For this review, take the finished solid that the model builds, in its own axes (mm). A direction names the side the tool comes from. Coordinates: 2 decimals unless noted, no trailing zeros. Loops run counter-clockwise (first coordinate to the right, second up) from the corner with the lowest first, then second, coordinate; pieces in that order, holes last. Notation, with made-up numbers: (-28, 48) -> (-7, 48) arc R23 cw to (-7, 83) -> close; hole circle Ø8 at (1.5, 75.25). An arc over 180 degrees is marked (long way). Answer in a Markdown table with one row per item.
from build123d import *

# Parameters (mm, degrees)
SKETCH1_W                 = 45
SKETCH1_H                 = 12.2
BASE_EXTRUDE_DEPTH        = 50
SKETCH16_W                = 33
SKETCH16_H                = 100
TABLE_EXTENSION_DEPTH     = 12.2
SKETCH3_R                 = 2.5
MOUNTHOLES_DEPTH          = 8
SKETCH14_W                = 2.9
SKETCH14_H                = 28.5
CONNECTION_DEPTH          = 44
SKETCH15_R                = 9.95
PISTON_DEPTH              = 72
SKETCH17_W                = 9
SKETCH17_H                = 0.5
SKETCH17_W_2              = 18
GROOVES_DEPTH             = 138.879557948
ENDLOCKPLATE1_DEPTH       = 9
ENDLOCKPLATE2_DEPTH       = 8
SKETCH20_R                = 2
ENDLOCKHOLES_DEPTH        = 117.232751409
SKETCH21_R                = 1.5
ENDLOCKADJUSTSCREWS_DEPTH = 2
SKETCH23_R                = 2
ENDLOCKMOUNTSCREWS_DEPTH  = 2
CHAMFER1_SIZE             = 0.3


with BuildPart() as part:
    # Sketch1 → Base-Extrude (new, symmetric)
    with BuildSketch(Plane.XY):
        Rectangle(SKETCH1_W, SKETCH1_H)
    extrude(amount=BASE_EXTRUDE_DEPTH, both=True)

    # Sketch16 → Table_Extension (add)
    with BuildSketch(Plane(origin=(0, 6.1, 0), x_dir=(-1, 0, 0), z_dir=(0, 1, 0))):
        with Locations((39, 0)):
            Rectangle(SKETCH16_W, SKETCH16_H)
    extrude(amount=-TABLE_EXTENSION_DEPTH)

    # Sketch3 → MountHoles (cut)
    with BuildSketch(Plane(origin=(0, 6.1, 0), x_dir=(-1, 0, 0), z_dir=(0, 1, 0))):
        with Locations(Location((32, -25, 0), (0, 0, 90))):
            Circle(SKETCH3_R)
        with Locations(Location((-8, -25, 0), (0, 0, 270))):
            Circle(SKETCH3_R)
        with Locations(Location((32, 25, 0), (0, 0, 270))):
            Circle(SKETCH3_R)
        with Locations(Location((-8, 25, 0), (0, 0, 90))):
            Circle(SKETCH3_R)
    extrude(amount=-MOUNTHOLES_DEPTH, mode=Mode.SUBTRACT)

    # Sketch14 → Connection (add, symmetric)
    with BuildSketch(Plane.XY):
        with Locations((0, -8.15)):
            Rectangle(SKETCH14_W, SKETCH14_H)
    extrude(amount=CONNECTION_DEPTH, both=True)

    # Sketch15 → Piston (add, symmetric)
    with BuildSketch(Plane.XY):
        with Locations((0, -22.4)):
            Circle(SKETCH15_R)
    extrude(amount=PISTON_DEPTH, both=True)

    # Sketch17 → Grooves (cut, through all)
    with BuildSketch(Plane.XY.offset(50)):
        with Locations((-51, 5.85)):
            Rectangle(SKETCH17_W, SKETCH17_H)
        with Locations((-13.5, 5.85)):
            Rectangle(SKETCH17_W_2, SKETCH17_H)
    extrude(amount=-GROOVES_DEPTH, mode=Mode.SUBTRACT)

    # Sketch18 → EndLockPlate1 (add, symmetric)
    with BuildSketch(Plane(origin=(-39, 0, 0), x_dir=(0, 0, -1), z_dir=(1, 0, 0))):
        Polygon((-50, 5.8), (-52, 5.8), (-52, -1.4), (-78, -1.4), (-78, -3.4), (-50, -3.4), align=None)
    endlockplate1 = extrude(amount=ENDLOCKPLATE1_DEPTH, both=True)

    # Sketch19 → EndLockPlate2 (add, symmetric)
    with BuildSketch(Plane(origin=(-39, 0, 0), x_dir=(0, 0, -1), z_dir=(1, 0, 0))):
        Polygon((-58, -1.4), (-58, -0.4), (-97, -0.4), (-97, -4.5), (-95.6, -5.9), (-78, -5.9), (-78, -1.4), align=None)
    endlockplate2 = extrude(amount=ENDLOCKPLATE2_DEPTH, both=True)

    # Sketch20 → EndLockHoles (cut, through all)
    with BuildSketch(Plane(origin=(0, -0.4, 0), x_dir=(-1, 0, 0), z_dir=(0, 1, 0))):
        with Locations(Location((39, 87.5, 0), (0, 0, 90))):
            Circle(SKETCH20_R)
        with BuildLine():
            Line((32.8, 63), (32.8, 69))
            ThreePointArc((32.8, 69), (33.8, 70), (34.8, 69))
            Line((34.8, 69), (34.8, 63))
            ThreePointArc((34.8, 63), (33.8, 62), (32.8, 63))
        make_face()
        with BuildLine():
            Line((43.2, 69), (43.2, 63))
            ThreePointArc((43.2, 63), (44.2, 62), (45.2, 63))
            Line((45.2, 63), (45.2, 69))
            ThreePointArc((45.2, 69), (44.2, 70), (43.2, 69))
        make_face()
    endlockholes = extrude(amount=-ENDLOCKHOLES_DEPTH, mode=Mode.SUBTRACT)

    # Sketch21 → EndLockAdjustScrews (add)
    with BuildSketch(Plane(origin=(0, -0.4, 0), x_dir=(-1, 0, 0), z_dir=(0, 1, 0))):
        with Locations(Location((44.2, 69, 0), (0, 0, 228.189685104))):
            Circle(SKETCH21_R)
        with Locations(Location((33.8, 69, 0), (0, 0, 228.189685104))):
            Circle(SKETCH21_R)
    endlockadjustscrews = extrude(amount=ENDLOCKADJUSTSCREWS_DEPTH)

    # Sketch23 → EndLockMountScrews (add)
    with BuildSketch(Plane.XY.offset(52)):
        with Locations(Location((-44.2, 2.7, 0), (0, 0, 180))):
            Circle(SKETCH23_R)
        with Locations(Location((-33.8, 2.7, 0), (0, 0, 180))):
            Circle(SKETCH23_R)
    endlockmountscrews = extrude(amount=ENDLOCKMOUNTSCREWS_DEPTH)

    # EndLockMirror: EndLockPlate1, EndLockPlate2, EndLockHoles, EndLockAdjustScrews, EndLockMountScrews across plane
    add(endlockplate1.mirror(Plane.XY))
    add(endlockplate2.mirror(Plane.XY))
    add(endlockholes.mirror(Plane.XY), mode=Mode.SUBTRACT)
    add(endlockadjustscrews.mirror(Plane.XY))
    add(endlockmountscrews.mirror(Plane.XY))

    # Chamfer1
    chamfer1_edges = [part.edges().sort_by_distance(p)[0] for p in [
        (-39, -0.4, 85.5),
        (-45.2, 1.6, 70.118033989),
        (-34.8, 1.6, 70.118033989),
        (-42.2, 2.7, 54),
        (-31.8, 2.7, 54),
        (-39, -0.4, -85.5),
        (-32, 6.1, -27.5),
        (-45.2, 1.6, -70.118033989),
        (-34.8, 1.6, -70.118033989),
        (8, 6.1, -22.5),
        (-32, 6.1, 27.5),
        (8, 6.1, 22.5),
    ]]
    chamfer(chamfer1_edges, length=CHAMFER1_SIZE)


solid = part.part
Item 1: Take a section at B-B, the plane x = -39. Count the separate pieces of the cut face and the enclosed holes in it, and give its area (3 significant figures).
Worked answers:
| item | result |
|---|---|
| separate pieces | 3 |
| enclosed holes | 0 |
| area | 1,560 mm² |
Item 2: For faces 1 (the cylindrical face through (-29.52, 2, -25.33)), 2 (the flat face through (-1.45, -9, 1)), 3 (the flat face through (-39, 2, 52)), 4 (the flat face through (-39, -2, -97)), 5 (the flat face through (-55.5, 0, -1)), list the 3-axis set-ups (+Z, -Z, +X, -X, +Y, -Y) from which the entire face can be reached by the end or side of a thin tool; tool diameter is ignored.
Worked answers:
| item | result |
|---|---|
| face 1 | +Y |
| face 2 | +Z, -Z, -X |
| face 3 | none |
| face 4 | -Z, +X, -X, +Y, -Y |
| face 5 | +Z, -Z, -X, +Y, -Y |
Item 3: Insertion check: pin 1 (5 mm diameter, centred on y = -11, z = 61.5, fed in from +X); pin 2 (0.5 mm diameter, centred on x = -30.5, y = -2.5, fed in from -Z); pin 3 (2 mm diameter, centred on x = -42.5, y = 1.5, fed in from -Z); pin 4 (6 mm diameter, centred on x = -5.5, z = -77.5, fed in from -Y). Each pin has a flat end and moves straight along its axis. Give the tip position at first contact, or say it passes through.
Worked answers:
| item | result |
|---|---|
| pin 1 | x = 4.45 |
| pin 2 | z = -78 |
| pin 3 | z = -70.32 |
| pin 4 | through |
Item 4: Take a section at C-C, the plane z = 48. State the section outline as (x, y) points.
Worked answers:
| item | result |
|---|---|
| outline | (-55.5, -6.1) -> (22.5, -6.1) -> (22.5, 6.1) -> (-4.5, 6.1) -> (-4.5, 5.6) -> (-22.5, 5.6) -> (-22.5, 6.1) -> (-46.5, 6.1) -> (-46.5, 5.6) -> (-55.5, 5.6) -> close; circle Ø19.9 at (0, -22.4) |
Item 5: Take a section at A-A, the plane z = -87.5. State the section outline as (x, y) points, and give its area (3 significant figures).
Worked answers:
| item | result |
|---|---|
| outline | (-47, -5.9) -> (-41, -5.9) -> (-41, -0.7) -> (-41.3, -0.4) -> (-47, -0.4) -> close; (-37, -5.9) -> (-31, -5.9) -> (-31, -0.4) -> (-36.7, -0.4) -> (-37, -0.7) -> close |
| area | 65.9 mm² |
Item 6: The part is to be moulded in two halves that separate along Y. For faces 6 (the flat face through (-39, -0.4, 77)), 7 (the cylindrical face through (-42.202, 2.612, 52.838)), 8 (the flat face through (-48, -2, -62)), say which applies: +Y half, -Y half, draft (parallel to the pull), parting line (faces both ways), or undercut.
Worked answers:
| item | result |
|---|---|
| face 6 | +Y half |
| face 7 | undercut |
| face 8 | draft |
Item 7: For L1, parallel to X at y = 0.5, z = 25; L2, parallel to Y at x = -27.5, z = 31; L3, parallel to Y at x = -18, z = -33, list the stretches that pass through material, from the lowest coordinate up.
Worked answers:
| item | result |
|---|---|
| L1 | -55.5 to -34.5, -29.5 to 5.5, 10.5 to 22.5 |
| L2 | -6.1 to 6.1 |
| L3 | -6.1 to 5.6 |
Item 8: Take a section at D-D, the plane z = -10. State the section outline as (x, y) points, and give its area (3 significant figures).
Worked answers:
| item | result |
|---|---|
| outline | (-55.5, -6.1) -> (-1.45, -6.1) -> (-1.45, -12.56) arc R9.95 ccw (long way) to (1.45, -12.56) -> (1.45, -6.1) -> (22.5, -6.1) -> (22.5, 6.1) -> (-4.5, 6.1) -> (-4.5, 5.6) -> (-22.5, 5.6) -> (-22.5, 6.1) -> (-46.5, 6.1) -> (-46.5, 5.6) -> (-55.5, 5.6) -> close |
| area | 1,270 mm² |
